Print and shaded views of the part. All mm, measured from the part's lowest x, y and z. Give positions to 0.01 mm unless a question says otherwise; leave off trailing zeros. Write each loop counter-clockwise with the first axis right and the second up, starting at its lowest first coordinate (ties: lowest second). Pieces come first, ordered by that corner, then holes. Notation, with made-up numbers: (22, 72) - (49, 72) arc R13 cw to (49, 88) - close; hole circle Ø7 at (-38, 23). An arc over 180 degrees is marked (long way). Use one line per item in the form item = value. Start each with the question number.
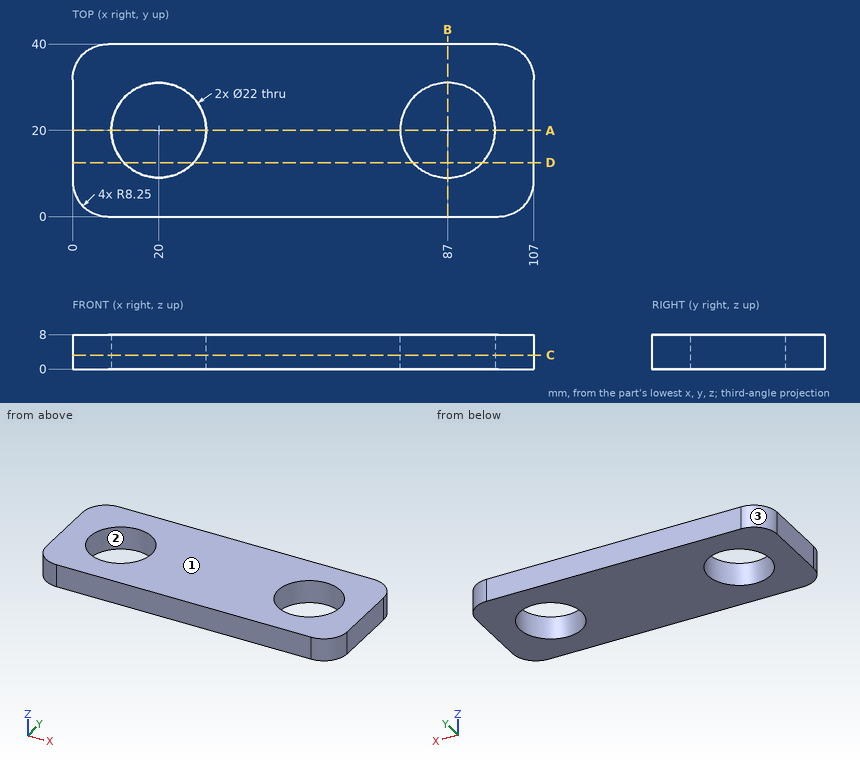
(1) Wall check: line 1 (Y direction, x = 20.5, z = 6); line 2 (X direction, y = 29.5, z = 2.75); line 3 (X direction, y = 15, z = 3). Give the ranges that are in metal, low to high. Write a range as from..to.
(2) Cut at B-B, the plane x = 87. Give the cut face in (y, z).
(3) Pin check, flat tips, straight feed: pin 1 Ø13 at (x, y) = (20, 20) entering from +Z; pin 2 Ø4 at (x, z) = (71.5, 2) entering from -Y; pin 3 Ø4 at (y, z) = (34, 2.5) entering from +X. Stop position of each tip, or through.
(4) Two-plate mould, pull along Y, no slides. Class the marked faces 1, 2 and 3: +Y half, -Y half, draft (parallel to the pull), parting line (faces both ways), or undercut.
(5) Cut at C-C, the plane z = 3.25. Give the cut face in (x, y).
(6) Cut at A-A, the plane y = 20. Give the cut face in (x, z), then the cut area to 3 significant figures.
(7) Cut at D-D, the plane y = 12.5. Give the cut face in (x, z), then the cut area to 3 significant figures.
Solution:
q1.line_1 = 0..9.01, 30.99..40
q1.line_2 = 0..14.45, 25.55..81.45, 92.55..107
q1.line_3 = 0..10.2, 29.8..77.2, 96.8..107
q2.outline = (0, 0) - (9, 0) - (9, 8) - (0, 8) - close; (31, 0) - (40, 0) - (40, 8) - (31, 8) - close
q3.pin_1 = through
q3.pin_2 = 0
q3.pin_3 = 107
q4.face_1 = draft
q4.face_2 = undercut
q4.face_3 = +Y half
q5.outline = (0, 8.25) arc R8.25 ccw to (8.25, 0) - (98.75, 0) arc R8.25 ccw to (107, 8.25) - (107, 31.75) arc R8.25 ccw to (98.75, 40) - (8.25, 40) arc R8.25 ccw to (0, 31.75) - close; hole circle Ø22 at (20, 20); hole circle Ø22 at (87, 20)
q6.outline = (0, 0) - (9, 0) - (9, 8) - (0, 8) - close; (31, 0) - (76, 0) - (76, 8) - (31, 8) - close; (98, 0) - (107, 0) - (107, 8) - (98, 8) - close
q6.area = 504 mm2
q7.outline = (0, 0) - (11.95, 0) - (11.95, 8) - (0, 8) - close; (28.05, 0) - (78.95, 0) - (78.95, 8) - (28.05, 8) - close; (95.05, 0) - (107, 0) - (107, 8) - (95.05, 8) - close
q7.area = 599 mm2
